from build123d import *
from build123d.topology import SkipClean

# Parameters (mm, degrees)
SKETCH1_R           = 20
SKETCH1_R_2         = 1
BOSS_EXTRUDE1_DEPTH = 3
BOSS_EXTRUDE2_DEPTH = 3
BOSS_EXTRUDE3_START = -2
BOSS_EXTRUDE3_DEPTH = 2
SKETCH4_R           = 1.5
CUT_EXTRUDE1_DEPTH  = 2
CHAMFER2_SIZE       = 1


with BuildPart() as part:
    # Sketch1 → Boss-Extrude1 (new body)
    with BuildSketch(Plane(origin=(0, 0, 0), x_dir=(1, 0, 0), z_dir=(0, 1, 0))):
        with Locations(Location((0, 0, 0), (0, 0, 270))):
            Circle(SKETCH1_R)
        with Locations(Location((-7.8, 7.8, 0), (0, 0, 270))):
            Circle(SKETCH1_R_2, mode=Mode.SUBTRACT)
        with Locations(Location((7.8, 7.8, 0), (0, 0, 270))):
            Circle(SKETCH1_R_2, mode=Mode.SUBTRACT)
        with Locations(Location((7.8, -7.8, 0), (0, 0, 270))):
            Circle(SKETCH1_R_2, mode=Mode.SUBTRACT)
        with Locations(Location((-7.8, -7.8, 0), (0, 0, 270))):
            Circle(SKETCH1_R_2, mode=Mode.SUBTRACT)
    extrude(amount=BOSS_EXTRUDE1_DEPTH)

    # Sketch2 → Boss-Extrude2 (add)
    with SkipClean():  # the faces are left unmerged after this step: merging them gives an invalid solid
        with BuildSketch(Plane(origin=(0, 3, 0), x_dir=(1, 0, 0), z_dir=(0, 1, 0))):
            with BuildLine():
                Line((-10.926328273, 13.985062443), (-12.313229507, 15.760215072))
                ThreePointArc((-12.313229507, 15.760215072), (-14.142135624, 14.142135624), (-15.760215072, 12.313229507))
                Line((-15.760215072, 12.313229507), (-13.985062443, 10.926328273))
                ThreePointArc((-13.985062443, 10.926328273), (-12.549235456, 12.549235456), (-10.926328273, 13.985062443))
            make_face()
            with BuildLine():
                Line((10.926328273, 13.985062443), (12.313229507, 15.760215072))
                ThreePointArc((12.313229507, 15.760215072), (14.142135624, 14.142135624), (15.760215072, 12.313229507))
                Line((15.760215072, 12.313229507), (13.985062443, 10.926328273))
                ThreePointArc((13.985062443, 10.926328273), (12.549235456, 12.549235456), (10.926328273, 13.985062443))
            make_face()
            with BuildLine():
                Line((13.985062443, -10.926328273), (15.760215072, -12.313229507))
                ThreePointArc((15.760215072, -12.313229507), (14.142135624, -14.142135624), (12.313229507, -15.760215072))
                Line((12.313229507, -15.760215072), (10.926328273, -13.985062443))
                ThreePointArc((10.926328273, -13.985062443), (12.549235456, -12.549235456), (13.985062443, -10.926328273))
            make_face()
            with BuildLine():
                Line((-10.926328273, -13.985062443), (-12.313229507, -15.760215072))
                ThreePointArc((-12.313229507, -15.760215072), (-14.142135624, -14.142135624), (-15.760215072, -12.313229507))
                Line((-15.760215072, -12.313229507), (-13.985062443, -10.926328273))
                ThreePointArc((-13.985062443, -10.926328273), (-12.549235456, -12.549235456), (-10.926328273, -13.985062443))
            make_face()
        extrude(amount=BOSS_EXTRUDE2_DEPTH)

    # Sketch3 → Boss-Extrude3 (add)
    with SkipClean():  # the faces are left unmerged after this step: merging them gives an invalid solid
        with BuildSketch(Plane(origin=(0, 6, 0), x_dir=(1, 0, 0), z_dir=(0, 1, 0)).offset(BOSS_EXTRUDE3_START)):
            with BuildLine():
                Line((12.313229507, 15.760215072), (16.007198358, 20.488279594))
                ThreePointArc((16.007198358, 20.488279594), (18.384776311, 18.384776311), (20.488279594, 16.007198358))
                Line((20.488279594, 16.007198358), (15.760215072, 12.313229507))
                ThreePointArc((15.760215072, 12.313229507), (14.142135624, 14.142135624), (12.313229507, 15.760215072))
            make_face()
            with BuildLine():
                Line((-12.313229507, 15.760215072), (-16.007198358, 20.488279594))
                ThreePointArc((-16.007198358, 20.488279594), (-18.384776311, 18.384776311), (-20.488279594, 16.007198358))
                Line((-20.488279594, 16.007198358), (-15.760215072, 12.313229507))
                ThreePointArc((-15.760215072, 12.313229507), (-14.142135624, 14.142135624), (-12.313229507, 15.760215072))
            make_face()
            with BuildLine():
                Line((15.760215072, -12.313229507), (20.488279594, -16.007198358))
                ThreePointArc((20.488279594, -16.007198358), (18.384776311, -18.384776311), (16.007198358, -20.488279594))
                Line((16.007198358, -20.488279594), (12.313229507, -15.760215072))
                ThreePointArc((12.313229507, -15.760215072), (14.142135624, -14.142135624), (15.760215072, -12.313229507))
            make_face()
            with BuildLine():
                Line((-12.313229507, -15.760215072), (-16.007198358, -20.488279594))
                ThreePointArc((-16.007198358, -20.488279594), (-18.384776311, -18.384776311), (-20.488279594, -16.007198358))
                Line((-20.488279594, -16.007198358), (-15.760215072, -12.313229507))
                ThreePointArc((-15.760215072, -12.313229507), (-14.142135624, -14.142135624), (-12.313229507, -15.760215072))
            make_face()
        extrude(amount=BOSS_EXTRUDE3_DEPTH)

    # Sketch4 → Cut-Extrude1 (cut)
    with SkipClean():  # the faces are left unmerged after this step: merging them gives an invalid solid
        with BuildSketch(Plane.XZ.offset(-4)):
            with Locations(Location((-16.263455967, -16.263455967, 0), (0, 0, 270))):
                Circle(SKETCH4_R)
            with Locations(Location((-16.263455967, 16.263455967, 0), (0, 0, 270))):
                Circle(SKETCH4_R)
            with Locations(Location((16.263455967, 16.263455967, 0), (0, 0, 270))):
                Circle(SKETCH4_R)
            with Locations(Location((16.263455967, -16.263455967, 0), (0, 0, 270))):
                Circle(SKETCH4_R)
        extrude(amount=-CUT_EXTRUDE1_DEPTH, mode=Mode.SUBTRACT)

    # Chamfer2
    # the kernel refuses this chamfer: 1 mm, written as the material it takes off along each edge
    with BuildSketch(Plane(origin=(-16.007198358, 1.428317012, 20.488279594), x_dir=(0.615661475325629, 0, -0.788010753606745), z_dir=(0, 1, 0)), Plane(origin=(20.488279594, 1.428317012, 16.007198358), x_dir=(-0.7880107536067236, 0, -0.6156614753256563), z_dir=(0, 1, 0)), Plane(origin=(16.007198358, 1.428317012, -20.488279594), x_dir=(-0.6156614753256462, 0, 0.7880107536067315), z_dir=(0, 1, 0)), Plane(origin=(-20.488279594, 1.428317012, -16.007198358), x_dir=(0.7880107536067239, 0, 0.6156614753256557), z_dir=(0, 1, 0))) as chamfer2_piece_1:
        with BuildLine():
            Line((CHAMFER2_SIZE, 0), (0.018531237, 0.981468763))
            ThreePointArc((0.018531237, 0.981468763), (0.004898706, 0.504686734), (0, 0))
            Line((0, 0), (CHAMFER2_SIZE, 0))
        make_face()
    extrude(amount=7.143365976, mode=Mode.SUBTRACT)
    with BuildSketch(Plane(origin=(-20.488279594, 1.428317012, 16.007198358), x_dir=(0.7880107536066959, 0, -0.6156614753256917), z_dir=(0, 1, 0)), Plane(origin=(16.007198358, 1.428317012, 20.488279594), x_dir=(-0.6156614753256615, 0, -0.7880107536067196), z_dir=(0, 1, 0)), Plane(origin=(20.488279594, 1.428317012, -16.007198358), x_dir=(-0.7880107536067122, 0, 0.615661475325671), z_dir=(0, 1, 0)), Plane(origin=(-16.007198358, 1.428317012, -20.488279594), x_dir=(0.615661475325662, 0, 0.7880107536067191), z_dir=(0, 1, 0))) as chamfer2_piece_2:
        with BuildLine():
            Line((CHAMFER2_SIZE, 0), (0.018531237, -0.981468763))
            ThreePointArc((0.018531237, -0.981468763), (0.004898706, -0.504686734), (0, 0))
            Line((0, 0), (CHAMFER2_SIZE, 0))
        make_face()
    extrude(amount=7.143365976, mode=Mode.SUBTRACT)


solid = part.part
Design review of the part built by this model. Coordinates are the model's own, in mm. A direction names the side the tool comes from. Round coordinates to 2 decimals unless told otherwise and drop trailing zeros. Write each loop counter-clockwise with the first axis right and the second up, starting at its lowest first coordinate (ties: lowest second). Pieces come first, ordered by that corner, then holes. Notation, with made-up numbers: (-16, 24) -> (31, 24) arc R34 ccw to (31, 56) -> close; hole circle Ø1 at (-24.5, 83). An arc over 180 degrees is marked (long way). One line per item, written item: value. Start each with the question number.
Q1. Add section B-B (y = 0.5). Give the boundary of the cut face in (x, z), then the cut area to 3 significant figures.
Q2. Add section A-A (z = 7.8). Give the boundary of the cut face in (x, y).
Q3. Insertion check: P1, Ø5, axis at x = 16.26, z = -16.26, coming from the +Y side; P2, Ø2.5, axis at x = -16.26, z = -16.26, coming from the -Y side; P3, Ø2, axis at x = 9, z = 10.5, coming from the +Y side; P4, Ø4, axis at x = 17, z = 15, coming from the -Y side. Each pin has a flat end and moves straight along its axis. Give the tip position at first contact, or say it passes through.
Q4. The part is to be moulded in two halves that separate along X. For faces 5 (the face through (18.36, 4.99, -18.41)), 6 (the face through (-19.784, 4.986, -16.071)), 7 (the face through (16.071, 4.986, -19.784)), say which applies: pulls with the +X half, pulls with the -X half, needs draft (parallel to the pull), parting line crosses it, or undercut.
Q5. Add section D-D (x = 13). Give the boundary of the cut face in (y, z), then the cut area to 3 significant figures.
Q6. Tool access review of faces 1 (the face through (19.784, 4.986, 16.071)), 2 (the face through (-16, 4, -18)), 3 (the face through (-16.071, 4.986, 19.784)), 4 (the face through (0, 3, 0)): name each direction out of +Z, -Z, +X, -X, +Y, -Y from which nothing blocks a thin tool from reaching the whole face with its end or side.
Q7. To check wall thickness, follow probe 1 along X at (y, z) = (2, 7.8); probe 2 along X at (y, z) = (5.7, -16.5); probe 3 along Z at (x, y) = (8, 1.85). State the ranges of each line that lie inside material, in increasing order.
Q8. Add section C-C (x = 7.8). Give the boundary of the cut face in (y, z).
Response:
1. outline: circle Ø40 at (0, 0); hole circle Ø2 at (-7.8, -7.8); hole circle Ø2 at (-7.8, 7.8); hole circle Ø2 at (7.8, -7.8); hole circle Ø2 at (7.8, 7.8)
1. area: 1,240 mm^2
2. outline: (-18.42, 0) -> (-8.8, 0) -> (-8.8, 3) -> (-18.42, 3) -> close; (-6.8, 0) -> (6.8, 0) -> (6.8, 3) -> (-6.8, 3) -> close; (8.8, 0) -> (18.42, 0) -> (18.42, 3) -> (8.8, 3) -> close
3. P1: stops at y = 6
3. P2: passes through
3. P3: stops at y = 3
3. P4: stops at y = 4
4. face 5: pulls with the +X half
4. face 6: pulls with the -X half
4. face 7: undercut
5. outline: (0, -15.2) -> (4, -15.2) -> (4, -16.64) -> (6, -16.64) -> (6, -12.08) -> (3, -12.08) -> (3, 12.08) -> (6, 12.08) -> (6, 16.64) -> (4, 16.64) -> (4, 15.2) -> (0, 15.2) -> close
5. area: 116 mm^2
6. face 1: +X, +Y, -Y
6. face 2: -Z, -X, -Y
6. face 3: +Z, +Y, -Y
6. face 4: +Y
7. probe 1: x = -18.42 to -8.8, -6.8 to 6.8, 8.8 to 18.42
7. probe 2: x = -19.84 to -17.74, -14.78 to -12.89, 12.89 to 14.78, 17.74 to 19.84
7. probe 3: z = -18.33 to -8.78, -6.82 to 6.82, 8.78 to 18.33
8. outline: (0, -18.42) -> (3, -18.42) -> (3, -8.8) -> (0, -8.8) -> close; (0, -6.8) -> (3, -6.8) -> (3, 6.8) -> (0, 6.8) -> close; (0, 8.8) -> (3, 8.8) -> (3, 18.42) -> (0, 18.42) -> close
